```python
from build123d import *

# Parameters (mm, degrees)
CROQUIS1_R                 = 18.75
SALIENTE_EXTRUIR1_DEPTH    = 1600
CROQUIS3_W                 = 8.15
CROQUIS3_H                 = 30
CORTAR_EXTRUIR1_DEPTH      = 5.75
CORTAR_EXTRUIR2_DEPTH      = 1601.219711477
CORTAR_EXTRUIR2_DEPTH_BACK = 1601.219711477
CROQUIS5_R                 = 4.7625
CORTAR_EXTRUIR3_DEPTH      = 1601.219711579
CORTAR_EXTRUIR3_DEPTH_BACK = 1601.219711579
CROQUIS6_R                 = 4.7625


with BuildPart() as part:
    # Croquis1 → Saliente-Extruir1 (new body)
    with BuildSketch(Plane(origin=(0, 0, 0), x_dir=(1, 0, 0), z_dir=(0, 1, 0))):
        with Locations(Location((0, 0, 0), (0, 0, 270))):
            Circle(CROQUIS1_R)
    extrude(amount=SALIENTE_EXTRUIR1_DEPTH)

    # Croquis3 → Cortar-Extruir1 (cut)
    with BuildSketch(Plane.XY.offset(18.75)):
        with Locations((0, 261.062165694)):
            Rectangle(CROQUIS3_W, CROQUIS3_H)
    cortar_extruir1 = extrude(amount=-CORTAR_EXTRUIR1_DEPTH, mode=Mode.SUBTRACT)

    # Simetría1: Cortar-Extruir1 across plane
    add(cortar_extruir1.mirror(Plane.XY), mode=Mode.SUBTRACT)

    # Croquis5 → Cortar-Extruir2 (cut, two sides: drawn at the far end of the back side and taken through both)
    with BuildSketch(Plane(origin=(0, 0, 0), x_dir=(0, 0, -1), z_dir=(1, 0, 0)).offset(-CORTAR_EXTRUIR2_DEPTH_BACK)):
        with Locations((0, 273.56)):
            Circle(CROQUIS5_R)
    extrude(amount=CORTAR_EXTRUIR2_DEPTH + CORTAR_EXTRUIR2_DEPTH_BACK, mode=Mode.SUBTRACT)

    # Croquis6 → Cortar-Extruir3 (cut, two sides: drawn at the far end of the back side and taken through both)
    with BuildSketch(Plane(origin=(0, 0, 0), x_dir=(0, 0, -1), z_dir=(1, 0, 0)).offset(-CORTAR_EXTRUIR3_DEPTH_BACK)):
        with Locations((0, 1338.56)):
            Circle(CROQUIS6_R)
    extrude(amount=CORTAR_EXTRUIR3_DEPTH + CORTAR_EXTRUIR3_DEPTH_BACK, mode=Mode.SUBTRACT)


solid = part.part
```
Here's how the part is built. I have some questions about the finished solid (model axes, mm). Coordinates: 2 decimals unless noted, no trailing zeros. Loops run counter-clockwise (first coordinate to the right, second up) from the corner with the lowest first, then second, coordinate; pieces in that order, holes last. Notation, with made-up numbers: (74.25, -8) - (103.25, -8) arc R22 ccw to (103.25, 7) - close; hole circle Ø10 at (75, 29.5). An arc over 180 degrees is marked (long way). Return JSON: item names as keys, results as strings. Group by question number.
Item 1: If we section it at A-A on y = 790.5: Write out the boundary of the cut face in (x, z).
Item 2: Will these pins go through, and if not, where does the flat tip stop? P1, Ø12, axis at y = 935, z = -9, coming from the -X side; P2, Ø2, axis at x = -4, y = 183, coming from the -Z side; P3, Ø4, axis at x = 0, y = 265, coming from the +Z side.
Item 3: I need wall thicknesses on line 1 (Y direction, x = -10.5, z = 0); line 2 (Y direction, x = 7.5, z = -1); line 3 (Z direction, x = 5, y = 1141.5). Which ranges of each line are inside material? Lowest first, please. Write a range as from..to.
Calculated:
{
 "1": {"outline": "circle Ø37.5 at (0, 0)"},
 "2": {"P1": "stops at x = -18.51", "P2": "stops at z = -18.51", "P3": "stops at z = 13"},
 "3": {"line 1": "y = 0..268.8, 278.32..1333.8, 1343.32..1600", "line 2": "y = 0..268.9, 278.22..1333.9, 1343.22..1600", "line 3": "z = -18.07..18.07"}
}
